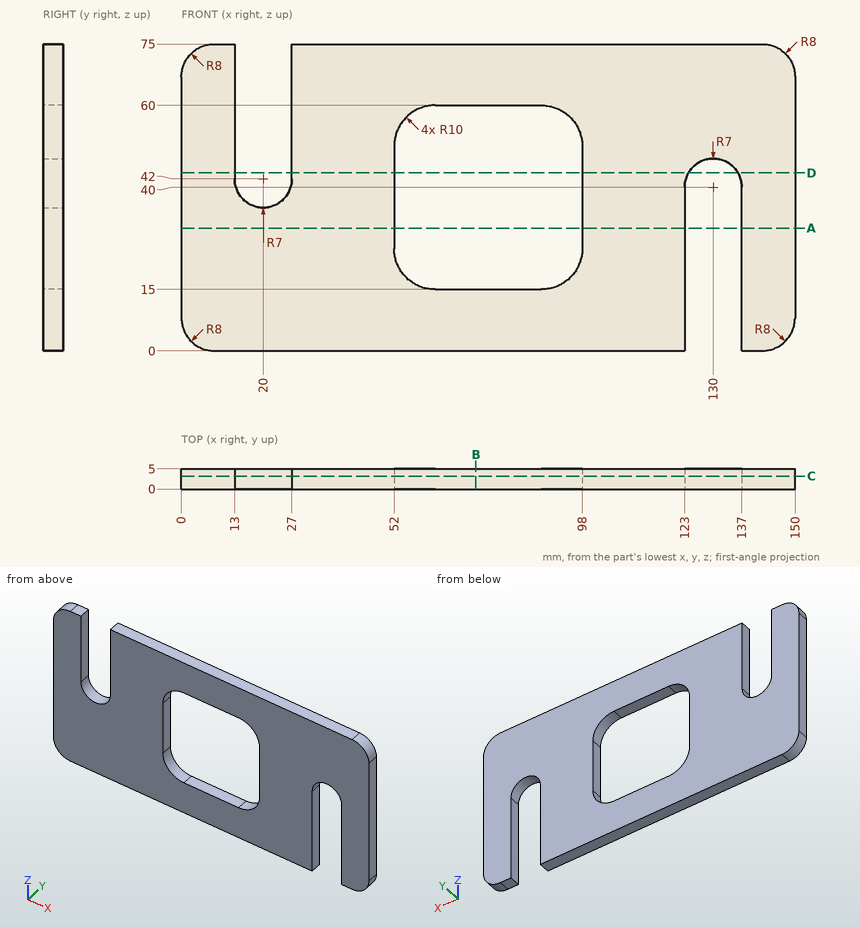
Could you check a few things on this drawing? It's one solid part, dimensions in mm from its lowest x, y, z. Round coordinates to 2 decimals unless told otherwise and drop trailing zeros. Order: outer loops, then holes, each group sorted by start corner. A loop starts at its lowest first (then second) coordinate and runs counter-clockwise, first axis right, second up. Notation, with made-up numbers: (-16, -24.5) -> (37, -24.5) arc R10 ccw to (37, -19.5) -> close; hole circle Ø1 at (86.5, 73). An arc over 180 degrees is marked (long way). One line per question, with ' | ' between items.
Q1. If we section it at D-D on z = 43.5: Write out the boundary of the cut face in (x, y).
Computed values:
outline: (0, 0) -> (13, 0) -> (13, 5) -> (0, 5) -> close; (27, 0) -> (52, 0) -> (52, 5) -> (27, 5) -> close; (98, 0) -> (123.94, 0) -> (123.94, 5) -> (98, 5) -> close; (136.06, 0) -> (150, 0) -> (150, 5) -> (136.06, 5) -> close
Q2. If we section it at A-A on z = 30: Write out the boundary of the cut face in (x, y), plus the area to 3 significant figures.
Computed values:
outline: (0, 0) -> (52, 0) -> (52, 5) -> (0, 5) -> close; (98, 0) -> (123, 0) -> (123, 5) -> (98, 5) -> close; (137, 0) -> (150, 0) -> (150, 5) -> (137, 5) -> close | area: 450 mm²
Q3. If we section it at C-C on y = 3.2: Write out the boundary of the cut face in (x, z), plus the area to 3 significant figures.
Computed values:
outline: (0, 8) arc R8 ccw to (8, 0) -> (123, 0) -> (123, 40) arc R7 cw to (137, 40) -> (137, 0) -> (142, 0) arc R8 ccw to (150, 8) -> (150, 67) arc R8 ccw to (142, 75) -> (27, 75) -> (27, 42) arc R7 cw to (13, 42) -> (13, 75) -> (8, 75) arc R8 ccw to (0, 67) -> close; hole (52, 25) arc R10 ccw to (62, 15) -> (88, 15) arc R10 ccw to (98, 25) -> (98, 50) arc R10 ccw to (88, 60) -> (62, 60) arc R10 ccw to (52, 50) -> close | area: 8,030 mm²
Q4. If we section it at B-B on x = 72: Write out the boundary of the cut face in (y, z).
Computed values:
outline: (0, 0) -> (5, 0) -> (5, 15) -> (0, 15) -> close; (0, 60) -> (5, 60) -> (5, 75) -> (0, 75) -> close
Q5. I'm going to push a flat-ended pin straight in: pin 1 (2.5 mm diameter, centred on y = 2, z = 38, fed in from -X). Where does the tip first touch, or does it pass through?
Computed values:
pin 1: x = 0
Q6. If I drill on line 1 (Z direction, x = 79, y = 0.4); line 2 (X direction, y = 1.1, z = 28); line 3 (X direction, y = 4.3, z = 8.5), over which ranges is the centre line in solid material (lowest first)? Write a range as from..to.
Computed values:
line 1: 0..15, 60..75 | line 2: 0..52, 98..123, 137..150 | line 3: 0..123, 137..150
